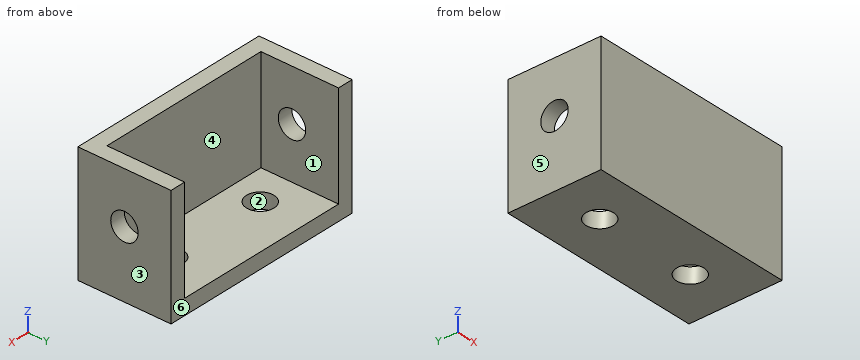
```python
from build123d import *

# Parameters (mm, degrees)
SKETCH_1_W          = 40
SKETCH_1_H          = 18
SKETCH_1_R          = 2.65
EXTRUDE_1_DEPTH     = 3
SKETCH_3_W          = 20
SKETCH_3_H          = 18
SKETCH_3_R          = 2.65
EXTRUDE_2_DEPTH     = 40
SKETCH_5_W          = 34
SKETCH_5_H          = 20
CUT_EXTRUDE_2_DEPTH = 15


with BuildPart() as part:
    # 草图1 → 凸台-拉伸1 (new body)
    with BuildSketch(Plane.XY):
        Rectangle(SKETCH_1_W, SKETCH_1_H)
        with Locations((-10, 0)):
            Circle(SKETCH_1_R, mode=Mode.SUBTRACT)
        with Locations((10, 0)):
            Circle(SKETCH_1_R, mode=Mode.SUBTRACT)
    extrude(amount=EXTRUDE_1_DEPTH)

    # 草图3 → 凸台-拉伸2 (add)
    with BuildSketch(Plane.ZY.offset(20)):
        with Locations((13, 0)):
            Rectangle(SKETCH_3_W, SKETCH_3_H)
        with Locations(Location((13, 0, 0), (0, 0, 270))):
            Circle(SKETCH_3_R, mode=Mode.SUBTRACT)
    extrude(amount=-EXTRUDE_2_DEPTH)

    # 草图5 → 切除-拉伸2 (cut)
    with BuildSketch(Plane(origin=(0, 9, 0), x_dir=(1, 0, 0), z_dir=(0, 1, 0))):
        with Locations((0, -13)):
            Rectangle(SKETCH_5_W, SKETCH_5_H)
    extrude(amount=-CUT_EXTRUDE_2_DEPTH, mode=Mode.SUBTRACT)


solid = part.part
```
Design review of the part built by this model. Coordinates are the model's own, in mm. Face numbers are marked on the shaded views. A direction names the side the tool comes from. Coordinates: 2 decimals unless noted, no trailing zeros. Loops run counter-clockwise (first coordinate to the right, second up) from the corner with the lowest first, then second, coordinate; pieces in that order, holes last.
Q1. We need section A-A on y = 0. State the section outline as (x, z) points.
Reported:
outline: (-20, 0) - (-12.65, 0) - (-12.65, 3) - (-17, 3) - (-17, 10.35) - (-20, 10.35) - close; (-20, 15.65) - (-17, 15.65) - (-17, 23) - (-20, 23) - close; (-7.35, 0) - (7.35, 0) - (7.35, 3) - (-7.35, 3) - close; (12.65, 0) - (20, 0) - (20, 10.35) - (17, 10.35) - (17, 3) - (12.65, 3) - close; (17, 15.65) - (20, 15.65) - (20, 23) - (17, 23) - close
Q2. Tool access review of the marked faces 1 and 2: name each direction out of +Z, -Z, +X, -X, +Y, -Y from which nothing blocks a thin tool from reaching the whole face with its end or side.
Reported:
face 1: +Z, +Y
face 2: +Z, -Z
Q3. We need section D-D on z = 4.25. State the section outline as (x, y) points.
Reported:
outline: (-20, -9) - (20, -9) - (20, 9) - (17, 9) - (17, -6) - (-17, -6) - (-17, 9) - (-20, 9) - close
Q4. To check wall thickness, follow line 1 (Z direction, x = -18.6, y = 0); line 2 (X direction, y = 1.75, z = 7); line 3 (Y direction, x = -10, z = 0.9). State the ranges of each line that lie inside material, in increasing order.
Reported:
line 1: z = 0 to 10.35, 15.65 to 23
line 2: x = -20 to -17, 17 to 20
line 3: y = -9 to -2.65, 2.65 to 9
Q5. We need section B-B on z = 13. State the section outline as (x, y) points.
Reported:
outline: (-20, -9) - (20, -9) - (20, -2.65) - (17, -2.65) - (17, -6) - (-17, -6) - (-17, -2.65) - (-20, -2.65) - close; (-20, 2.65) - (-17, 2.65) - (-17, 9) - (-20, 9) - close; (17, 2.65) - (20, 2.65) - (20, 9) - (17, 9) - close
Q6. We need section C-C on x = 10. State the section outline as (y, z) points, and give its area (3 significant figures).
Reported:
outline: (-9, 0) - (-2.65, 0) - (-2.65, 3) - (-6, 3) - (-6, 23) - (-9, 23) - close; (2.65, 0) - (9, 0) - (9, 3) - (2.65, 3) - close
area: 98.1 mm2
Q7. For pin 1 (6 mm diameter, centred on x = -6.5, z = 18, fed in from +Y); pin 2 (7.5 mm diameter, centred on x = -8, y = 2.5, fed in from +Z); pin 3 (7 mm diameter, centred on y = 0, z = 13, fed in from -X), all flat-tipped, find the tip position at first contact; note any pin that passes through.
Reported:
pin 1: stops at y = -6
pin 2: stops at z = 3
pin 3: stops at x = -20
Q8. The part is to be moulded in two halves that separate along X. For the marked faces 3, 4, 5 and 6, say which applies: +X half, -X half, draft (parallel to the pull), parting line (faces both ways), or undercut.
Reported:
face 3: +X half
face 4: undercut
face 5: -X half
face 6: draft
